```python
from build123d import *

# Parameters (mm, degrees)
SKETCH1_W           = 10
SKETCH1_H           = 10
BOSS_EXTRUDE1_DEPTH = 5
SKETCH2_R           = 2.5
CUT_EXTRUDE1_DEPTH  = 4
SKETCH3_R           = 1.755
CUT_EXTRUDE2_DEPTH  = 1
SKETCH4_R           = 2.57854844
BOSS_EXTRUDE2_DEPTH = 7
SKETCH5_R           = 1.755
BOSS_EXTRUDE3_DEPTH = 2.5
SKETCH6_W           = 4
SKETCH6_H           = 1
BOSS_EXTRUDE4_DEPTH = 1


with BuildPart() as part:
    # Sketch1 → Boss-Extrude1 (new body)
    with BuildSketch(Plane.XY):
        with Locations((5, 5)):
            Rectangle(SKETCH1_W, SKETCH1_H)
    extrude(amount=BOSS_EXTRUDE1_DEPTH)

    # Sketch2 → Cut-Extrude1 (cut)
    with BuildSketch(Plane(origin=(0, 0, 0), x_dir=(-1, 0, 0), z_dir=(0, 0, -1))):
        with Locations((-5, 5)):
            Circle(SKETCH2_R)
    extrude(amount=-CUT_EXTRUDE1_DEPTH, mode=Mode.SUBTRACT)

    # Sketch3 → Cut-Extrude2 (cut)
    with BuildSketch(Plane(origin=(0, 0, 4), x_dir=(-1, 0, 0), z_dir=(0, 0, -1))):
        with Locations((-5, 5)):
            Circle(SKETCH3_R)
    extrude(amount=-CUT_EXTRUDE2_DEPTH, mode=Mode.SUBTRACT)

    # Sketch4 → Boss-Extrude2 (add)
    with BuildSketch(Plane(origin=(0, 0, 4), x_dir=(-1, 0, 0), z_dir=(0, 0, -1))):
        with Locations((-5, 5.07854844)):
            Circle(SKETCH4_R)
    extrude(amount=BOSS_EXTRUDE2_DEPTH)

    # Sketch5 → Boss-Extrude3 (add)
    with BuildSketch(Plane.XY.offset(4)):
        with Locations(Location((5, 5, 0), (0, 0, 180))):
            Circle(SKETCH5_R)
    extrude(amount=BOSS_EXTRUDE3_DEPTH)

    # Sketch6 → Boss-Extrude4 (add)
    with BuildSketch(Plane.XY.offset(5)):
        with Locations((5, 9.5)):
            Rectangle(SKETCH6_W, SKETCH6_H)
    boss_extrude4 = extrude(amount=BOSS_EXTRUDE4_DEPTH)

    # Mirror1: Boss-Extrude4 across plane
    add(boss_extrude4.mirror(Plane(origin=(0, 5, 0), x_dir=(0, 0, 1), z_dir=(0, -1, 0))))


solid = part.part
```
Design review of the part built by this model. Coordinates are the model's own, in mm. A direction names the side the tool comes from. Round coordinates to 2 decimals unless told otherwise and drop trailing zeros. Order: outer loops, then holes, each group sorted by start corner. A loop starts at its lowest first (then second) coordinate and runs counter-clockwise, first axis right, second up. Notation, with made-up numbers: (-26, 87.25) - (-19, 87.25) arc R15 cw to (-19, 99.25) - close; hole circle Ø5 at (27.5, 76.25). An arc over 180 degrees is marked (long way). Return JSON: item names as keys, results as strings.
Q1. Machinability: for faces 1 (the flat face through (5, 9.5, 6)), 2 (the flat face through (3, 7, 0)), 3 (the flat face through (7, 0.5, 5.5)), which of the approach directions +Z, -Z, +X, -X, +Y, -Y give a long, thin tool a straight path to every point of the face, cutting with its end or side? Answer none if there is none.
Computed values:
{"face 1": "+Z, +X, -X, +Y", "face 2": "-Z", "face 3": "+Z, +X, +Y, -Y"}
Q2. The part is to be moulded in two halves that separate along Y. For faces 4 (the flat face through (3, 9.5, 5.5)), 5 (the cylindrical face through (2.54, 5.85, -1.48)), 6 (the flat face through (5, 0, 3)), 7 (the cylindrical face through (5.38, 6.713, 5.74)), say which applies: pulls with the +Y half, pulls with the -Y half, needs draft (parallel to the pull), parting line crosses it, or undercut.
Computed values:
{"face 4": "needs draft", "face 5": "parting line crosses it", "face 6": "pulls with the -Y half", "face 7": "undercut"}
Q3. Wall thickness on L1, parallel to Y at x = 5.5, z = 5.5; L2, parallel to Z at x = 7.25, y = 3.25; L3, parallel to Z at x = 4.25, y = 9.75: over which ranges is each line inside the solid? List them lowest first. Write a range as [from, to].
Computed values:
{"L1": "y = [0, 1], [3.32, 6.68], [9, 10]", "L2": "z = [0, 5]", "L3": "z = [0, 6]"}
Q4. For pin 1 Ø1.1 at (y, z) = (0.5, 5.5) entering from -X; pin 2 Ø0.5 at (y, z) = (9.5, 5.5) entering from -X; pin 3 Ø0.5 at (x, y) = (5.5, 0.5) entering from +Z, all flat-tipped, find the tip position at first contact; note any pin that passes through.
Computed values:
{"pin 1": "stops at x = 0", "pin 2": "stops at x = 3", "pin 3": "stops at z = 6"}
Q5. Consider section C-C on y = 6.5. Write out the cut boundary in (x, z), plus the area to 3 significant figures.
Computed values:
{"outline": "(0, 0) - (2.85, 0) - (2.85, -3) - (7.15, -3) - (7.15, 0) - (10, 0) - (10, 5) - (5.91, 5) - (5.91, 6.5) - (4.09, 6.5) - (4.09, 5) - (0, 5) - close", "area": "65.6 mm2"}
Q6. Consider section B-B on y = 4.75. Write out the cut boundary in (x, z).
Computed values:
{"outline": "(0, 0) - (2.44, 0) - (2.44, -3) - (7.56, -3) - (7.56, 0) - (10, 0) - (10, 5) - (6.74, 5) - (6.74, 6.5) - (3.26, 6.5) - (3.26, 5) - (0, 5) - close"}
Q7. Consider section A-A on x = 5. Write out the cut boundary in (y, z) (3 decimals), plus the area to 3 significant figures.
Computed values:
{"outline": "(0, 0) - (2.5, 0) - (2.5, -3) - (7.657, -3) - (7.657, 0) - (10, 0) - (10, 6) - (9, 6) - (9, 5) - (6.755, 5) - (6.755, 6.5) - (3.245, 6.5) - (3.245, 5) - (1, 5) - (1, 6) - (0, 6) - close", "area": "72.7 mm2"}
Q8. Consider section D-D on x = 1.5. Write out the cut boundary in (y, z), plus the area to 3 significant figures.
Computed values:
{"outline": "(0, 0) - (10, 0) - (10, 5) - (0, 5) - close", "area": "50.0 mm2"}
